```python
from build123d import *

# Parameters (mm, degrees)
SKETCH1_R                       = 60.96
BILLET_DEPTH                    = 5.842
SKETCH4_R                       = 0.7493
FIRST_KEROSENE_OUTLET_DEPTH     = 88.140881336
PRIMARY_HOLES_COUNT             = 6
SECOND_START                    = -5.842
SECOND_RING_OUTLINE_R           = 0.7493
SECOND_RING_DEPTH               = 5.842
THIRD_START                     = -5.842
THIRD_RING_OUTLINE_R            = 0.7493
THIRD_RING_DEPTH                = 5.842
SKETCH18_RX                     = 46.67504
SKETCH18_RY                     = 22.225
KEROSENE_WELL_DEPTH             = 2.032
SKETCH17_R                      = 6.35
BOSS_EXTRUDE1_DEPTH             = 2.54
BOSS_EXTRUDE1_DIRECTION_2_REACH = 88.408
SKETCH21_R                      = 6.35
CUT_EXTRUDE1_DEPTH              = 2.54
CUT_EXTRUDE2_DEPTH              = 2.032
F_1_8_0_125_DIAMETER_HOLE2_D    = 3.175
SKETCH31_R                      = 8.740396603
SKETCH31_R_2                    = 6.200396603
CUT_EXTRUDE4_DEPTH              = 1.778
SKETCH32_R                      = 55.7149
SKETCH32_R_2                    = 51.6509
CUT_EXTRUDE5_DEPTH              = 2.6924


# Read off the part's stored shape, not the designer's step: Second ring, Third Ring
with BuildPart() as part:
    # Sketch1 → Billet (new body)
    with BuildSketch(Plane(origin=(0, 0, 0), x_dir=(1, 0, 0), z_dir=(0, 1, 0))):
        with Locations(Location((0, 0, 0), (0, 0, 270))):
            Circle(SKETCH1_R)
    extrude(amount=-BILLET_DEPTH)

    # Sketch4 → First Kerosene Outlet (cut, symmetric)
    with BuildSketch(Plane(origin=(0, -12.7, 0), x_dir=(1, 0, 0), z_dir=(0, 1, 0))):
        with Locations(Location((8.9916, 0, 0), (0, 0, 270))):
            Circle(SKETCH4_R)
        with Locations(Location((13.4874, 0, 0), (0, 0, 270))):
            Circle(SKETCH4_R)
        with Locations(Location((17.9832, 0, 0), (0, 0, 270))):
            Circle(SKETCH4_R)
    first_kerosene_outlet = extrude(amount=FIRST_KEROSENE_OUTLET_DEPTH, both=True, mode=Mode.SUBTRACT)

    # Primary Holes: First Kerosene Outlet ×6 about axis
    primary_holes_axis = Axis((0, 0, 0), (0, 1, 0))
    for i in range(1, PRIMARY_HOLES_COUNT):
        add(first_kerosene_outlet.rotate(primary_holes_axis, i * 360 / PRIMARY_HOLES_COUNT), mode=Mode.SUBTRACT)

    # Second ring outline → Second ring (cut)
    with BuildSketch(Plane(origin=(0, 0, 0), x_dir=(1, 0, 0), z_dir=(0, 1, 0)).offset(SECOND_START)):
        with Locations((11.680431031, 6.7437)):
            Circle(SECOND_RING_OUTLINE_R)
        with Locations((0, 13.4874)):
            Circle(SECOND_RING_OUTLINE_R)
        with Locations((-11.680431031, 6.7437)):
            Circle(SECOND_RING_OUTLINE_R)
        with Locations((-11.680431031, -6.7437)):
            Circle(SECOND_RING_OUTLINE_R)
        with Locations((0, -13.4874)):
            Circle(SECOND_RING_OUTLINE_R)
        with Locations((11.680431031, -6.7437)):
            Circle(SECOND_RING_OUTLINE_R)
    extrude(amount=SECOND_RING_DEPTH, mode=Mode.SUBTRACT)

    # Third Ring outline → Third Ring (cut)
    with BuildSketch(Plane(origin=(0, 0, 0), x_dir=(1, 0, 0), z_dir=(0, 1, 0)).offset(THIRD_START)):
        with Locations((17.370437319, 4.654394652)):
            Circle(THIRD_RING_OUTLINE_R)
        with Locations((15.573908041, 8.9916)):
            Circle(THIRD_RING_OUTLINE_R)
        with Locations((12.716042667, 12.716042667)):
            Circle(THIRD_RING_OUTLINE_R)
        with Locations((4.654394652, 17.370437319)):
            Circle(THIRD_RING_OUTLINE_R)
        with Locations((0, 17.9832)):
            Circle(THIRD_RING_OUTLINE_R)
        with Locations((-4.654394652, 17.370437319)):
            Circle(THIRD_RING_OUTLINE_R)
        with Locations((-12.716042667, 12.716042667)):
            Circle(THIRD_RING_OUTLINE_R)
        with Locations((-15.573908041, 8.9916)):
            Circle(THIRD_RING_OUTLINE_R)
        with Locations((-17.370437319, 4.654394652)):
            Circle(THIRD_RING_OUTLINE_R)
        with Locations((-17.370437319, -4.654394652)):
            Circle(THIRD_RING_OUTLINE_R)
        with Locations((-15.573908041, -8.9916)):
            Circle(THIRD_RING_OUTLINE_R)
        with Locations((-12.716042667, -12.716042667)):
            Circle(THIRD_RING_OUTLINE_R)
        with Locations((-4.654394652, -17.370437319)):
            Circle(THIRD_RING_OUTLINE_R)
        with Locations((0, -17.9832)):
            Circle(THIRD_RING_OUTLINE_R)
        with Locations((4.654394652, -17.370437319)):
            Circle(THIRD_RING_OUTLINE_R)
        with Locations((12.716042667, -12.716042667)):
            Circle(THIRD_RING_OUTLINE_R)
        with Locations((15.573908041, -8.9916)):
            Circle(THIRD_RING_OUTLINE_R)
        with Locations((17.370437319, -4.654394652)):
            Circle(THIRD_RING_OUTLINE_R)
    extrude(amount=THIRD_RING_DEPTH, mode=Mode.SUBTRACT)

    # Sketch18 → Kerosene Well (cut)
    with BuildSketch(Plane(origin=(0, 0, 0), x_dir=(1, 0, 0), z_dir=(0, 1, 0))):
        with Locations(Location((0, 0), (0, 0, -180))):
            Ellipse(SKETCH18_RX, SKETCH18_RY)
    extrude(amount=-KEROSENE_WELL_DEPTH, mode=Mode.SUBTRACT)

    # Sketch17 → Boss-Extrude1 (add)
    with BuildSketch(Plane(origin=(0, 0, 0), x_dir=(1, 0, 0), z_dir=(0, 1, 0))):
        with Locations(Location((0, 0, 0), (0, 0, 270))):
            Circle(SKETCH17_R)
    extrude(amount=BOSS_EXTRUDE1_DEPTH)

    # Sketch17 → Boss-Extrude1 direction 2 (add, up to next)
    with BuildSketch(Plane(origin=(0, 0, 0), x_dir=(1, 0, 0), z_dir=(0, 1, 0)), mode=Mode.PRIVATE) as boss_extrude1_direction_2_sk1:
        with Locations(Location((0, 0, 0), (0, 0, 270))):
            Circle(SKETCH17_R)
    boss_extrude1_direction_2_tool1 = extrude(boss_extrude1_direction_2_sk1.sketch, amount=-BOSS_EXTRUDE1_DIRECTION_2_REACH, mode=Mode.PRIVATE) - part.part
    add(boss_extrude1_direction_2_tool1.solids().sort_by_distance((0, 0, 0))[0])

    # Sketch21 → Cut-Extrude1 (cut)
    with BuildSketch(Plane(origin=(0, 2.54, 0), x_dir=(1, 0, 0), z_dir=(0, 1, 0))):
        with Locations(Location((0, 0, 0), (0, 0, 270))):
            Circle(SKETCH21_R)
    extrude(amount=-CUT_EXTRUDE1_DEPTH, mode=Mode.SUBTRACT)

    # Sketch24 → Cut-Extrude2 (cut)
    with BuildSketch(Plane(origin=(0, 0, 0), x_dir=(1, 0, 0), z_dir=(0, 1, 0))):
        with BuildLine():
            Line((-15.732765962, 20.924382105), (-21.799630657, 31.4325))
            ThreePointArc((-21.799630657, 31.4325), (-20.6375, 35.769630657), (-16.300369343, 34.6075))
            Line((-16.300369343, 34.6075), (-8.915091663, 21.81582383))
            add(Edge.make_bspline(
                [(-8.915091663, 21.81582383), (-12.395027666, 21.493390748), (-15.732765962, 20.924382105)],
                knots=[4.904573252, 4.904573252, 4.904573252, 5.056192247, 5.056192247, 5.056192247], degree=2, weights=[1, 0.997127836, 1]))
        make_face()
    extrude(amount=-CUT_EXTRUDE2_DEPTH, mode=Mode.SUBTRACT)

    # 1/8 (0.125) Diameter Hole2 (through all)
    with Locations(Plane(origin=(19.05, 0, -33.02), x_dir=(0, 0, 1), z_dir=(0, 1, 0))):
        with Locations((0, 0)):
            Hole(F_1_8_0_125_DIAMETER_HOLE2_D / 2)

    # Sketch31 → Cut-Extrude4 (cut)
    with BuildSketch(Plane(origin=(0, 0, 0), x_dir=(1, 0, 0), z_dir=(0, 1, 0))):
        with Locations(Location((19.05, 33.02, 0), (0, 0, 270))):
            Circle(SKETCH31_R)
        with Locations(Location((19.05, 33.02, 0), (0, 0, 270))):
            Circle(SKETCH31_R_2, mode=Mode.SUBTRACT)
    extrude(amount=-CUT_EXTRUDE4_DEPTH, mode=Mode.SUBTRACT)

    # Sketch32 → Cut-Extrude5 (cut)
    with BuildSketch(Plane.XZ.offset(5.842)):
        with Locations(Location((0, 0, 0), (0, 0, 270))):
            Circle(SKETCH32_R)
        with Locations(Location((0, 0, 0), (0, 0, 270))):
            Circle(SKETCH32_R_2, mode=Mode.SUBTRACT)
    extrude(amount=-CUT_EXTRUDE5_DEPTH, mode=Mode.SUBTRACT)


solid = part.part
```
Input: part model. Units: mm. Frame: model coordinates. A direction names the side the tool comes from. Round coordinates to 2 decimals unless told otherwise and drop trailing zeros. Order: outer loops, then holes, each group sorted by start corner. A loop starts at its lowest first (then second) coordinate and runs counter-clockwise, first axis right, second up. Notation, with made-up numbers: (84, -4.75) - (115, -4.75) arc R17 cw to (115, 24.25) - close; hole circle Ø1 at (13.5, 82). An arc over 180 degrees is marked (long way). Answer in a Markdown table with one row per item.
Item 1: Section query A-A (z = -33.02). Return the cut outline in (x, y) (1 decimal), then the cut area to 3 significant figures.
Model answer:
| item | result |
|---|---|
| outline | (-51.2, -5.8) - (-44.9, -5.8) - (-44.9, -3.1) - (-39.7, -3.1) - (-39.7, -5.8) - (17.5, -5.8) - (17.5, 0) - (12.8, 0) - (12.8, -1.8) - (10.3, -1.8) - (10.3, 0) - (-15.4, 0) - (-15.4, -2) - (-22.2, -2) - (-22.2, 0) - (-51.2, 0) - close; (20.6, -5.8) - (39.7, -5.8) - (39.7, -3.1) - (44.9, -3.1) - (44.9, -5.8) - (51.2, -5.8) - (51.2, 0) - (27.8, 0) - (27.8, -1.8) - (25.3, -1.8) - (25.3, 0) - (20.6, 0) - close |
| area | 529 mm² |
Item 2: Pin query (flat end, axial travel): pin 1 (1.3 mm diameter, centred on x = -11.68, z = -6.74, fed in from +Y); pin 2 (2 mm diameter, centred on y = -5, z = 22.5, fed in from -X); pin 3 (2.5 mm diameter, centred on x = -12.72, z = 12.72, fed in from +Y); pin 4 (2 mm diameter, centred on x = 35, y = -3, fed in from +Z). Return the tip coordinate at first contact, or that it passes through.
Model answer:
| item | result |
|---|---|
| pin 1 | passes through |
| pin 2 | stops at x = -57.04 |
| pin 3 | stops at y = -2.03 |
| pin 4 | stops at z = 50.6 |
Item 3: Reachability of faces 1 (the cylindrical face through (51.21, -4.51, 6.72)), 2 (the cylindrical face through (10.517, -0.877, -34.915)), 3 (the flat face through (-49, -5.842, 27)) from +Z, -Z, +X, -X, +Y, -Y: full face, straight path, thin tool, end or side. Return the list, or none.
Model answer:
| item | result |
|---|---|
| face 1 | -Y |
| face 2 | +Y |
| face 3 | +Z, -Z, +X, -X, -Y |
Item 4: Section query B-B (y = -4.95). Give the number of separate pieces and of enclosed holes in the cut face, then the cut area to 3 significant figures.
Model answer:
| item | result |
|---|---|
| separate pieces | 2 |
| enclosed holes | 44 |
| area | 10,200 mm² |
Item 5: Mould query, pull axis X, two halves, no side actions, for faces 4 (the cylindrical face through (60.44, -2.88, -7.94)), 5 (the flat face through (1, 0, 26)), 6 (the cylindrical face through (19.527, -2.962, -34.534)). Classes: released by +X, released by -X, zero draft, split by the parting line, or undercut.
Model answer:
| item | result |
|---|---|
| face 4 | split by the parting line |
| face 5 | zero draft |
| face 6 | undercut |
Item 6: Section query C-C (z = 47.5). Return the cut outline in (x, y).
Model answer:
| item | result |
|---|---|
| outline | (-38.21, -5.84) - (-29.12, -5.84) - (-29.12, -3.15) - (-20.29, -3.15) - (-20.29, -5.84) - (20.29, -5.84) - (20.29, -3.15) - (29.12, -3.15) - (29.12, -5.84) - (38.21, -5.84) - (38.21, 0) - (-38.21, 0) - close |
Item 7: Line query: line 1 (Z direction, x = -17, y = -5.05); line 2 (Z direction, x = 22, y = -0.9); line 3 (X direction, y = -5.6, z = 9.5). Output: solid intervals per line, ascending.
Model answer:
| item | result |
|---|---|
| line 1 | z = -58.54 to -53.06, -48.77 to -5.31, -4 to 4, 5.31 to 48.77, 53.06 to 58.54 |
| line 2 | z = -56.85 to -41.25, -38.47 to -27.57, -24.79 to -19.6, 19.6 to 56.85 |
| line 3 | x = -60.22 to -54.9, -50.77 to -16.12, -15.02 to 15.02, 16.12 to 50.77, 54.9 to 60.22 |
